from build123d import *

# Parameters (mm, degrees)
F0_W     = 60
F0_H     = 80
F0_R     = 20
F0_R_2   = 10
F0_R_3   = 5
F1_DEPTH = 6.35
F2_DEPTH = 12.7


# Not quite as in the source:
# - a feature names something its author has since deleted; it is built from what else it names


with BuildPart() as f1:
    # F0 (on Front) → F1 (new body)
    with BuildSketch(Plane.XZ):
        Rectangle(F0_W, F0_H)
        with Locations((0, -16.8533538189)):
            Circle(F0_R, mode=Mode.SUBTRACT)
        with Locations((0, 13.3463527084)):
            Circle(F0_R_2, mode=Mode.SUBTRACT)
        with Locations((0, 31.2290439901)):
            Circle(F0_R_3, mode=Mode.SUBTRACT)
    extrude(amount=F1_DEPTH)

    # F0 (on Front) → F2 (join)
    with BuildSketch(Plane.XZ):
        with Locations((0, -16.8533538189)):
            Circle(F0_R)
    extrude(amount=F2_DEPTH)


solid = f1.part
Geometry check sheet. Reference: the model listing, model coordinates, mm. A direction names the side the tool comes from. Round coordinates to 2 decimals unless told otherwise and drop trailing zeros. Loops run counter-clockwise (first coordinate to the right, second up) from the corner with the lowest first, then second, coordinate; pieces in that order, holes last. Notation, with made-up numbers: (59, -25) - (118, -25) arc R25 ccw to (118, 7) - close; hole circle Ø2 at (24.25, -10). An arc over 180 degrees is marked (long way). Answer as CSV lines item,"result".
(1) Cross-section at A-A, the plane x = 0. Enter the section's corners in (y, z), and give its area (4 significant figures).
Output values:
outline,"(-12.7, -36.85) - (-6.35, -36.85) - (-6.35, -40) - (0, -40) - (0, 3.35) - (-6.35, 3.35) - (-6.35, 3.15) - (-12.7, 3.15) - close; (-6.35, 23.35) - (0, 23.35) - (0, 26.23) - (-6.35, 26.23) - close; (-6.35, 36.23) - (0, 36.23) - (0, 40) - (-6.35, 40) - close"
area,"571.5 mm²"
(2) Material ranges on line 1 along Z through (x, y) = (0, -3.75); line 2 along X through (y, z) = (-2, 31); line 3 along Z through (x, y) = (4.5, -5.25), recorded low to high.
Output values:
line 1,"z = -40 to 3.35, 23.35 to 26.23, 36.23 to 40"
line 2,"x = -30 to -4.99, 4.99 to 30"
line 3,"z = -40 to 4.42, 22.28 to 29.05, 33.41 to 40"
(3) Set-up check for faces 1 (the face through (-4.336, -9.481, -36.378)), 2 (the face through (0, -3, 40)): record each of +Z, -Z, +X, -X, +Y, -Y from which the full face is reachable in a straight line by a thin tool's end or side.
Output values:
face 1,"-Y"
face 2,"+Z, +X, -X, +Y, -Y"
(4) Cross-section at D-D, the plane z = -27. Enter the section's corners in (x, y), and give its area (3 significant figures).
Output values:
outline,"(-30, -6.35) - (-17.24, -6.35) - (-17.24, -12.7) - (17.24, -12.7) - (17.24, -6.35) - (30, -6.35) - (30, 0) - (-30, 0) - close"
area,"600 mm²"
(5) Cross-section at B-B, the plane z = 9. Enter the section's corners in (x, y), and give its area (3 significant figures).
Output values:
outline,"(-30, -6.35) - (-9.01, -6.35) - (-9.01, 0) - (-30, 0) - close; (9.01, -6.35) - (30, -6.35) - (30, 0) - (9.01, 0) - close"
area,"267 mm²"
(6) Cross-section at C-C, the plane y = -1.5. Enter the section's corners in (x, z).
Output values:
outline,"(-30, -40) - (30, -40) - (30, 40) - (-30, 40) - close; hole circle Ø20 at (0, 13.35); hole circle Ø10 at (0, 31.23)"
(7) Release check for a two-part mould opening along X. For faces 3 (the face through (30, -3, -1)), 4 (the face through (-0.651, -3.131, 36.186)), 5 (the face through (0, 0, 1)) record: released by +X, released by -X, zero draft, split by the parting line, or undercut.
Output values:
face 3,"released by +X"
face 4,"undercut"
face 5,"zero draft"
